Could you check a few things on this model? Use its own coordinates, in mm. Coordinates: 2 decimals unless noted, no trailing zeros. Write each loop counter-clockwise with the first axis right and the second up, starting at its lowest first coordinate (ties: lowest second). Pieces come first, ordered by that corner, then holes.
Item 1: I want a section at C-C on x = -113. Please give me the cut outline in (y, z), then the cut area to 3 significant figures.
Item 2: If I drill on probe 1 along X at (y, z) = (1.35, 6.5); probe 2 along X at (y, z) = (0.95, 82) (3 decimals); probe 3 along Z at (x, y) = (-108.5, 0.35), over which ranges is the centre line in solid material (lowest first)?
Item 3: Thinking about a two-plate mould opening in Z: for faces 1 (the cylindrical face through (-133.025, 0.74, 67.423)), 2 (the cylindrical face through (-127.395, 0.761, 79.583)), 3 (the cylindrical face through (-129.61, 0.74, 51.59)), which applies, +Z half, -Z half, draft (parallel to the pull), parting line (faces both ways), or undercut?
Item 4: I want a section at A-A on y = 0.3. State how many separate pieces and enclosed holes the cut face has, then the cut area to 3 significant figures.
Item 5: I want a section at B-B on z = 45. Please give me the cut outline in (x, y).
Item 6: For P1, Ø2.5, axis at x = -132.45, z = 66.04, coming from the +Y side, with a flat end and sliding along its axis, tell me the tip position at first contact or that it passes through.
from build123d import *

# Parameters (mm, degrees)
ESQUISSE1_R             = 1.5
BOSS_EXTRU_1_DEPTH      = 1.5
ENL_V_MAT_EXTRU_1_DEPTH = 189.733992158
CONG_1_R                = 5
CONG_2_R                = 2


with BuildPart() as part:
    # Esquisse1 → Boss.-Extru.1 (new body)
    with BuildSketch(Plane(origin=(0, 0, 0), x_dir=(1, 0, 0), z_dir=(0, 1, 0))):
        with BuildLine():
            Line((-155, 0), (-139.5, 0))
            ThreePointArc((-139.5, 0), (-129.342147712, -52.257619782), (-100.347902147, -96.904842679))
            Line((-100.347902147, -96.904842679), (-111.497669052, -107.672047421))
            ThreePointArc((-111.497669052, -107.672047421), (-143.713497458, -58.064021979), (-155, 0))
        make_face()
        with Locations(Location((-146.374347778, -21.875792847, 0), (0, 0, 270))):
            Circle(ESQUISSE1_R, mode=Mode.SUBTRACT)
        with Locations(Location((-132.450285517, -66.03727634, 0), (0, 0, 270))):
            Circle(ESQUISSE1_R, mode=Mode.SUBTRACT)
    extrude(amount=BOSS_EXTRU_1_DEPTH)

    # Esquisse2 → Enlèv. mat.-Extru.1 (cut, through all)
    with BuildSketch(Plane(origin=(0, 1.5, 0), x_dir=(1, 0, 0), z_dir=(0, 1, 0))):
        with BuildLine():
            Line((-155, 0), (-144.5, 0))
            Line((-144.5, 0), (-154.217397717, -15.556164093))
            ThreePointArc((-154.217397717, -15.556164093), (-154.804225792, -7.78791865), (-155, 0))
        make_face()
        with BuildLine():
            Line((-106.461511638, -102.808686738), (-111.497669052, -107.672047421))
            ThreePointArc((-111.497669052, -107.672047421), (-129.740451706, -84.808108051), (-143.363022468, -58.924051021))
            ThreePointArc((-143.363022468, -58.924051021), (-125.74115641, -81.563361553), (-106.461511638, -102.808686738))
        make_face()
    extrude(amount=-ENL_V_MAT_EXTRU_1_DEPTH, mode=Mode.SUBTRACT)

    # Congé1
    cong_1_edges = [part.edges().sort_by_distance(p)[0] for p in [
        (-154.217397717, 0.75, 15.556164093),
        (-144.5, 0.75, 0),
        (-143.363022468, 0.75, 58.924051021),
        (-106.461511638, 0.75, 102.808686738),
    ]]
    fillet(cong_1_edges, radius=CONG_1_R)

    # Congé2
    cong_2_edges = [part.edges().sort_by_distance(p)[0] for p in [
        (-100.347902147, 0.75, 96.904842679),
        (-139.5, 0.75, 0),
    ]]
    fillet(cong_2_edges, radius=CONG_2_R)


solid = part.part
Response values:
1. outline: (0, 81.8) - (1.5, 81.8) - (1.5, 95.96) - (0, 95.96) - close
1. area: 21.2 mm2
2. probe 1: x = -148.56 to -139.35
2. probe 2: x = -125.373 to -112.855
2. probe 3: z = 87.68 to 100.25
3. face 1: undercut
3. face 2: +Z half
3. face 3: -Z half
4. separate pieces: 1
4. enclosed holes: 2
4. area: 1,380 mm2
5. outline: (-148.32, 0) - (-132.04, 0) - (-132.04, 1.5) - (-148.32, 1.5) - close
6. P1: passes through
